from build123d import *

# Parameters (mm, degrees)
F1_DEPTH = 26.8
F2_R     = 5


with BuildPart() as f1:
    # F0 (on Top) → F1 (new body)
    with BuildSketch(Plane.XY):
        Polygon((55.8652869582, 39.3723181486), (-11.5347130418, 39.3723181486), (-11.5347130418, 12.5723181486), (-38.3347130418, 12.5723181486), (-38.3347130418, -54.8276818514), (-11.5347130418, -54.8276818514), (-11.5347130418, -81.6276818514), (55.8652869582, -81.6276818514), (55.8652869582, -54.8276818514), (82.6652869582, -54.8276818514), (82.6652869582, 12.5723181486), (55.8652869582, 12.5723181486), align=None)
    extrude(amount=F1_DEPTH)

    # F2
    f2_edges = [f1.edges().sort_by_distance(p)[0] for p in [
        (-11.534713, -68.227682, 26.8),
        (22.165287, -81.627682, 26.8),
        (55.865287, -68.227682, 26.8),
        (69.265287, -54.827682, 26.8),
        (82.665287, -21.127682, 26.8),
        (69.265287, 12.572318, 26.8),
        (55.865287, 25.972318, 26.8),
        (22.165287, 39.372318, 26.8),
        (-11.534713, 25.972318, 26.8),
        (-24.934713, 12.572318, 26.8),
        (-38.334713, -21.127682, 26.8),
        (-24.934713, -54.827682, 26.8),
        (55.865287, -81.627682, 13.4),
        (55.865287, -54.827682, 13.4),
        (82.665287, -54.827682, 13.4),
        (82.665287, 12.572318, 13.4),
        (82.665287, -21.127682, 0),
        (-11.534713, -81.627682, 13.4),
        (22.165287, -81.627682, 0),
        (-11.534713, -54.827682, 13.4),
        (69.265287, -54.827682, 0),
        (-38.334713, 12.572318, 13.4),
        (-38.334713, -54.827682, 13.4),
        (-38.334713, -21.127682, 0),
        (-11.534713, 39.372318, 13.4),
        (-11.534713, 12.572318, 13.4),
        (-11.534713, 25.972318, 0),
        (55.865287, 39.372318, 13.4),
        (22.165287, 39.372318, 0),
        (55.865287, -68.227682, 0),
        (-24.934713, 12.572318, 0),
    ]]
    fillet(f2_edges, radius=F2_R)


solid = f1.part
Work out the finished part from the listing and answer in its coordinate system (mm). A direction names the side the tool comes from. Coordinates: 2 decimals unless noted, no trailing zeros. Order: outer loops, then holes, each group sorted by start corner. A loop starts at its lowest first (then second) coordinate and runs counter-clockwise, first axis right, second up. Notation, with made-up numbers: (42, -28) - (58, -28) arc R32 cw to (58, 8) - close; hole circle Ø3 at (51, 3.25). An arc over 180 degrees is marked (long way). Put each result on its own line as item: value. Start each with the question number.
1) Find the intervals of material crossed by line 1 (Y direction, x = -21.5, z = 10.5); line 2 (X direction, y = -76, z = 15.5); line 3 (X direction, y = 8, z = 15), in increasing order. Write a range as from..to.
2) Find section A-A (y = 19.5). Give the vertices of the cut face in (x, z).
3) Flat-ended cylindrical pins translate along their axes: pin 1 (4 mm diameter, centred on x = 70, z = 12, fed in from +Y); pin 2 (8.5 mm diameter, centred on y = -67, z = 11, fed in from -X); pin 3 (11 mm diameter, centred on y = 27, z = 7.5, fed in from +X). Find the tip coordinate at first contact, or state that the pin passes through.
4) Find section D-D (z = 3.25). Give the vertices of the cut face in (x, y), plus the area to 3 significant figures.
5) Find section C-C (x = -26). Give the vertices of the cut face in (y, z), plus the area to 3 significant figures.
6) Find section B-B (z = 18.25). Give the vertices of the cut face in (x, y).
7) For faces 1 (the cylindrical face through (-25.052, 11.147, 1.504)), 2 (the flat face through (-25, -54.828, 11)), 3 (the flat face through (67, 12.572, 11)), 4 (the cylindrical face through (69.4, -53.4, 25.3)), 5 (the cylindrical face through (-10.109, 25.855, 25.296)), determine the directions among +Z, -Z, +X, -X, +Y, -Y from which every point of the face is accessible in a straight line to the end or side of a thin tool.
Results list:
1. line 1: y = -54.83..12.57
1. line 2: x = -11.53..55.87
1. line 3: x = -38.32..82.65
2. outline: (-11.53, 5) arc R5 ccw to (-6.53, 0) - (55.87, 0) - (55.87, 21.8) arc R5 ccw to (50.87, 26.8) - (-6.53, 26.8) arc R5 ccw to (-11.53, 21.8) - close
3. pin 1: stops at y = 12.57
3. pin 2: stops at x = -11.53
3. pin 3: stops at x = 55.87
4. outline: (-38.02, -51.58) arc R5 ccw to (-33.33, -54.83) - (-16.53, -54.83) arc R5 cw to (-11.53, -59.83) - (-11.53, -76.63) arc R5 ccw to (-8.28, -81.31) - (50.87, -81.31) arc R4.68 ccw to (55.55, -76.63) - (55.55, -59.83) arc R5.32 cw to (60.87, -54.51) - (77.67, -54.51) arc R4.68 ccw to (82.35, -49.83) - (82.35, 9.32) arc R5 ccw to (77.67, 12.57) - (55.87, 12.57) - (55.87, 34.37) arc R5 ccw to (52.62, 39.06) - (-6.53, 39.06) arc R4.68 ccw to (-11.22, 34.37) - (-11.22, 17.57) arc R5.32 cw to (-16.53, 12.26) - (-33.33, 12.26) arc R4.68 ccw to (-38.02, 7.57) - close
4. area: 11,600 mm^2
5. outline: (-54.83, 0) - (7.57, 0) arc R5 ccw to (12.57, 5) - (12.57, 21.8) arc R5 ccw to (7.57, 26.8) - (-49.83, 26.8) arc R5 ccw to (-54.83, 21.8) - close
5. area: 1,790 mm^2
6. outline: (-38.33, -49.83) arc R5 ccw to (-33.33, -54.83) - (-16.53, -54.83) arc R5 cw to (-11.53, -59.83) - (-11.53, -76.63) arc R5 ccw to (-6.53, -81.63) - (50.87, -81.63) arc R5 ccw to (55.87, -76.63) - (55.87, -59.83) arc R5 cw to (60.87, -54.83) - (77.67, -54.83) arc R5 ccw to (82.67, -49.83) - (82.67, 7.57) arc R5 ccw to (77.67, 12.57) - (55.87, 12.57) - (55.87, 34.37) arc R5 ccw to (50.87, 39.37) - (-6.53, 39.37) arc R5 ccw to (-11.53, 34.37) - (-11.53, 17.57) arc R5 cw to (-16.53, 12.57) - (-33.33, 12.57) arc R5 ccw to (-38.33, 7.57) - close
7. face 1: -Z, -X, +Y
7. face 2: +Z, -Z, -X, -Y
7. face 3: +Z, -Z, +X, +Y
7. face 4: +Z, +X, -Y
7. face 5: +Z, -X, +Y
